The figure shows three views and two pictorial views of one solid part (mm, origin at its lowest corner). Answer the questions. A direction names the side the tool comes from. Coordinates: 2 decimals unless noted, no trailing zeros. Order: outer loops, then holes, each group sorted by start corner. A loop starts at its lowest first (then second) coordinate and runs counter-clockwise, first axis right, second up.
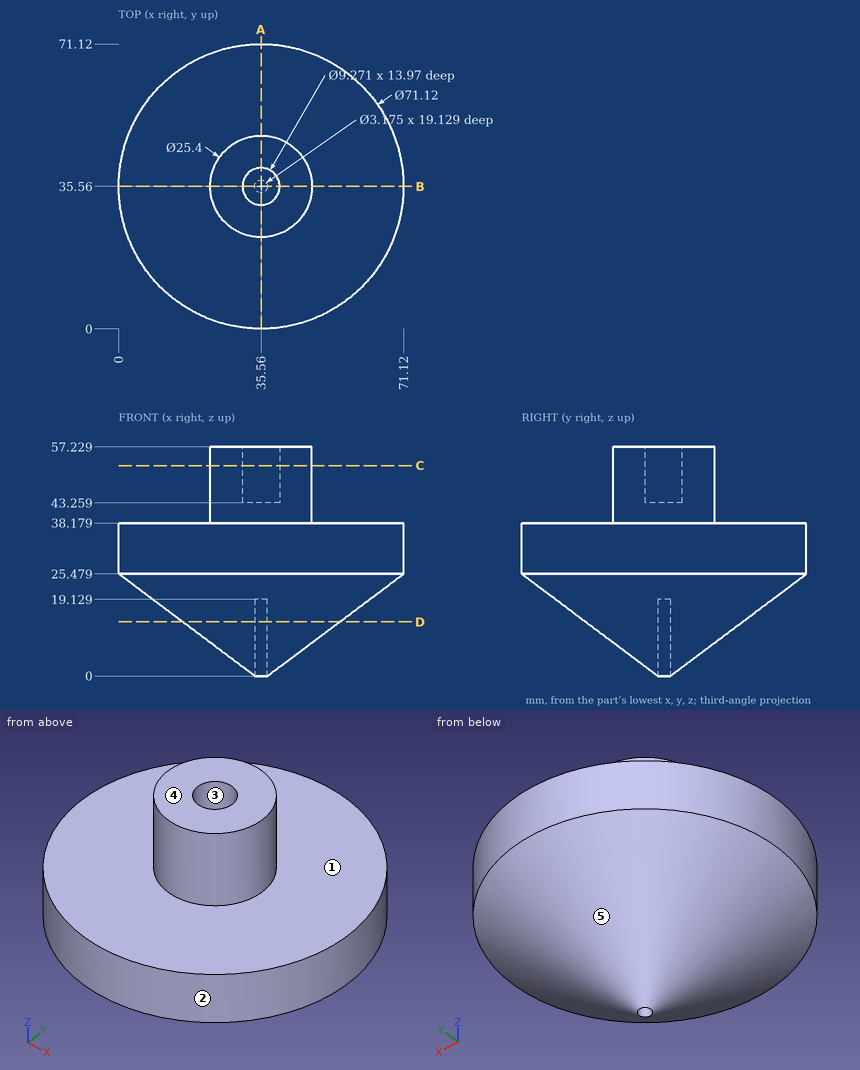
1) For the marked faces 1 and 2, determine the directions among +Z, -Z, +X, -X, +Y, -Y from which every point of the face is accessible in a straight line to the end or side of a thin tool.
2) Straight lines are drawn through the part: probe 1 along Y at (x, z) = (35.56, 53.25) (1 decimal); probe 2 along X at (y, z) = (35, 5) (1 decimal); probe 3 along Z at (x, y) = (59, 36). For each, find the intervals that lie inside material, in ascending order.
3) The mould has two halves that part along X. Classify the marked faces 3, 4 and 5: released by +X, released by -X, zero draft, split by the parting line, or undercut.
4) A cutting plane is placed at D-D, the plane z = 13.5. Write down the section's boundary in (x, y) (1 decimal), plus the area to 3 significant figures.
5) A cutting plane is placed at C-C, the plane z = 52.5. Write down the section's boundary in (x, y) (1 decimal).
6) A cutting plane is placed at A-A, the plane x = 35.56. Write down the section's boundary in (y, z) (1 decimal), plus the area to 3 significant figures.
7) Each of these flat-tipped pins is pushed along its axis until it touches: P1, Ø3.5, axis at x = 36, y = 36, coming from the -Z side; P2, Ø3, axis at x = 49.5, z = 33, coming from the +Y side; P3, Ø12, axis at x = 48.5, z = 11.5, coming from the +Y side; P4, Ø10, axis at x = 48, z = 50, coming from the +Y side. Where does it stop, or does it pass through?
Working result:
1. face 1: +Z
1. face 2: +Z, -Z
2. probe 1: y = 22.9 to 30.9, 40.2 to 48.3
2. probe 2: x = 27.3 to 34.1, 37 to 43.8
2. probe 3: z = 16.39 to 38.18
3. face 3: undercut
3. face 4: zero draft
3. face 5: split by the parting line
4. outline: circle Ø39.2 at (35.6, 35.6); hole circle Ø3.2 at (35.6, 35.6)
4. area: 1,200 mm2
5. outline: circle Ø25.4 at (35.6, 35.6); hole circle Ø9.3 at (35.6, 35.6)
6. outline: (0, 25.5) - (34, 0) - (34, 19.1) - (37.1, 19.1) - (37.1, 0) - (71.1, 25.5) - (71.1, 38.2) - (48.3, 38.2) - (48.3, 57.2) - (40.2, 57.2) - (40.2, 43.3) - (30.9, 43.3) - (30.9, 57.2) - (22.9, 57.2) - (22.9, 38.2) - (0, 38.2) - close
6. area: 2,140 mm2
7. P1: stops at z = 0
7. P2: stops at y = 68.87
7. P3: stops at y = 57.44
7. P4: stops at y = 45.85
